Autodesk Fusion 360 part; units mm, degrees
sketch "Sketch1" plane through (0, 0, 0) normal (0, 1, 0) x (1, 0, 0)
  circle A0 centre (0, 0) radius 11.75
  circle A1 centre (0, 0) radius 30
  circle A2 centre (0, 0) radius 20.5
  dimension "d1" = 23.5
  dimension "d2" = 60
  dimension "d3" = 41
extrude "Extrude1" add sketch "Sketch1" along normal blind 2 contours A1 | A2
extrude "Extrude2" add sketch "Sketch1" along normal blind 5 contours A1
chamfer "Chamfer1" distance 2 angle 45 1 edges at (-19.1127, 5, -7.4131)
Geometry check sheet. Reference: the model listing, model coordinates, mm. A direction names the side the tool comes from. Round coordinates to 2 decimals unless told otherwise and drop trailing zeros. Write each loop counter-clockwise with the first axis right and the second up, starting at its lowest first coordinate (ties: lowest second). Pieces come first, ordered by that corner, then holes. Notation, with made-up numbers: (45, -19.75) -> (91, -19.75) arc R29 cw to (91, 12.25) -> close; hole circle Ø10 at (65.5, 27.5). An arc over 180 degrees is marked (long way). One line per item, written item: value. Start each with the question number.
(1) Cross-section at B-B, the plane z = 0. Record the cut outline in (x, y), and give its area (3 significant figures).
(2) Cross-section at A-A, the plane x = 0. Record the cut outline in (y, z).
(3) Cross-section at D-D, the plane z = 23.5. Record the cut outline in (x, y), and give its area (3 significant figures).
(4) Scan lines: line 1 (X direction, y = 1.3, z = 0); line 2 (X direction, y = 2.4, z = 0). Record each from-to range of solid material in increasing order. Write a range as [from, to].
(5) Go/stop test with flat-tipped pins: pin 1 Ø2 at (x, y) = (22, 3.5) entering from +Z; pin 2 Ø1.5 at (x, z) = (-9, -3) entering from +Y; pin 3 Ø1 at (x, y) = (1, 3.5) entering from +Z; pin 4 Ø1 at (x, y) = (-5.5, 1.5) entering from -Z. Record where each tip stops, or that it passes through.
(6) Draft check along Z on faces 3 (the cylindrical face through (-29.97, 2.46, 1.32)), 4 (the cylindrical face through (11.207, 0.986, 3.529)), 5 (the flat face through (4.3, 5, -22.4)). Enter one of: +Z half, -Z half, draft (parallel to the pull), parting line (faces both ways), or undercut.
(7) Access from +Z, -Z, +X, -X, +Y, -Y to the whole of each face (thin tool, end or side, straight path). Record for faces 1 (the flat face through (9, 2, 9)), 2 (the flat face through (0, 0, 13)).
(8) Cross-section at C-C, the plane y = 1. Record the cut outline in (x, z), and give its area (3 significant figures).
Answer:
1. outline: (-30, 0) -> (-11.75, 0) -> (-11.75, 2) -> (-20.5, 2) -> (-20.5, 3) -> (-22.5, 5) -> (-30, 5) -> close; (11.75, 0) -> (30, 0) -> (30, 5) -> (22.5, 5) -> (20.5, 3) -> (20.5, 2) -> (11.75, 2) -> close
1. area: 126 mm²
2. outline: (0, -30) -> (5, -30) -> (5, -22.5) -> (3, -20.5) -> (2, -20.5) -> (2, -11.75) -> (0, -11.75) -> close; (0, 11.75) -> (2, 11.75) -> (2, 20.5) -> (3, 20.5) -> (5, 22.5) -> (5, 30) -> (0, 30) -> close
3. outline: (-18.65, 0) -> (18.65, 0) -> (18.65, 5) -> (-18.65, 5) -> close
3. area: 186 mm²
4. line 1: [-30, -11.75], [11.75, 30]
4. line 2: [-30, -20.5], [20.5, 30]
5. pin 1: z = 21.42
5. pin 2: through
5. pin 3: z = 30
5. pin 4: z = -29.58
6. face 3: parting line
6. face 4: undercut
6. face 5: draft
7. face 1: +Y
7. face 2: +Z, -Z, +X, -X, -Y
8. outline: circle Ø60 at (0, 0); hole circle Ø23.5 at (0, 0)
8. area: 2,390 mm²
